For this review, take the finished solid that the model builds, in its own axes (mm). A direction names the side the tool comes from. Coordinates: 2 decimals unless noted, no trailing zeros. Loops run counter-clockwise (first coordinate to the right, second up) from the corner with the lowest first, then second, coordinate; pieces in that order, holes last.
Autodesk Inventor part; units mm, degrees
sketch "Sketch1" plane through (0, 0, 0) normal (0, 0, 1) x (1, 0, 0)
  line L0 (0, 2.8582) -> (0, -2.8582) construction
  line L1 (-5.7775, 0) -> (5.7775, 0) construction
  line L2 (-18.15, -15.5) -> (18.15, -15.5)
  line L3 (18.15, -15.5) -> (18.15, 15.5)
  line L4 (18.15, 15.5) -> (-18.15, 15.5)
  line L5 (-18.15, 15.5) -> (-18.15, -15.5)
  line L6 (-18.15, -15.5) -> (18.15, 15.5) construction
  line L7 (18.15, -15.5) -> (-18.15, 15.5) construction
  point P0 (0, 0)
  point P1 (0, 0)
  dimension "d0" = 36.3
  dimension "d1" = 31
extrude "Extrusion1" add sketch "Sketch1" along normal blind 2.5
sketch "Sketch2" plane through (0, 0, 2.5) normal (0, 0, 1) x (1, 0, 0)
  line L0 (18.15, -15.5) -> (-18.15, -15.5)
  line L1 (-18.15, -15.5) -> (-18.15, 15.5)
  line L2 (-18.15, 15.5) -> (18.15, 15.5)
  line L3 (18.15, 15.5) -> (18.15, -15.5)
  line L4 (-18.15, 15.5) -> (-16.15, 15.5)
  line L5 (-16.15, 15.5) -> (-16.15, -15.5)
  line L6 (-16.15, -15.5) -> (-18.15, -15.5)
  line L7 (-18.15, -15.5) -> (-18.15, 15.5)
  point P0 (0, 0)
  dimension "d4" = 2
extrude "Extrusion2" add sketch "Sketch2" along normal blind 3.5 contours L0 L1 L2 L5
sketch "Sketch3" plane through (0, 0, 6) normal (0, 0, 1) x (1, 0, 0)
  line L0 (-16.15, 15.5) -> (-16.15, -15.5)
  line L1 (-16.15, -15.5) -> (-18.15, -15.5)
  line L2 (-18.15, -15.5) -> (-18.15, 15.5)
  line L3 (-18.15, 15.5) -> (-16.15, 15.5)
  line L4 (-18.15, 5) -> (11.85, 5)
  line L5 (11.85, 5) -> (11.85, -5)
  line L6 (11.85, -5) -> (-18.15, -5)
  line L7 (-18.15, -5) -> (-18.15, 5)
  line L8 (-25.41, 0) -> (25.41, 0)
  point P0 (0, 0)
  point P1 (-16.15, 5)
  point P2 (-16.15, -5)
  dimension "d7" = 10
  dimension "d8" = 5
  dimension "d9" = 30
extrude "Extrusion3" add sketch "Sketch3" along normal blind 2.5
sketch "Sketch4" plane through (0, 0, 2.5) normal (0, 0, 1) x (1, 0, 0)
  line L0 (-16.15, 15.5) -> (-16.15, -15.5)
  line L1 (18.15, -15.5) -> (-16.15, -15.5)
  line L2 (18.15, 15.5) -> (18.15, -15.5)
  line L3 (-16.15, 15.5) -> (18.15, 15.5)
  line L4 (-18.15, 15.5) -> (-16.15, 15.5)
  line L5 (-18.15, -15.5) -> (-18.15, 15.5)
  line L6 (-16.15, -15.5) -> (-18.15, -15.5)
  line L7 (-16.15, 15.5) -> (11.85, 15.5)
  line L8 (11.85, 15.5) -> (11.85, 13)
  line L9 (11.85, 13) -> (-16.15, 13)
  line L10 (-16.15, 13) -> (-16.15, 15.5)
  line L11 (-16.15, -15.5) -> (11.85, -15.5)
  line L12 (11.85, -15.5) -> (11.85, -13)
  line L13 (11.85, -13) -> (-16.15, -13)
  line L14 (-16.15, -13) -> (-16.15, -15.5)
  point P0 (18.15, 13.5)
  point P1 (11.85, -15.5)
  point P2 (11.85, 15.5)
  dimension "d16" = 2.5
  dimension "d17" = 6.3
  dimension "d18" = 6.3
  dimension "d19" = 2.5
extrude "Extrusion4" add sketch "Sketch4" along normal up to surface (6 mm away) contours L3 L8 L9 L0 | L13 L12 L1 L0
sketch "Sketch5" plane through (0, 0, 2.5) normal (0, 0, 1) x (1, 0, 0)
  line L0 (11.85, 13) -> (-16.15, 13)
  line L1 (-16.15, -13) -> (-16.15, 13)
  line L2 (-16.15, -13) -> (11.85, -13)
  line L3 (11.85, -13) -> (11.85, -15.5)
  line L4 (18.15, -15.5) -> (11.85, -15.5)
  line L5 (18.15, 15.5) -> (18.15, -15.5)
  line L6 (11.85, 15.5) -> (18.15, 15.5)
  line L7 (11.85, 15.5) -> (11.85, 13)
  line L8 (11.85, -15.5) -> (-18.15, -15.5)
  line L9 (-18.15, -15.5) -> (-18.15, 15.5)
  line L10 (-18.15, 15.5) -> (11.85, 15.5)
  line L11 (18.15, -15.5) -> (11.85, -15.5)
  line L12 (11.85, -15.5) -> (11.85, 15.5)
  line L13 (11.85, 15.5) -> (18.15, 15.5)
  line L14 (18.15, 15.5) -> (18.15, -15.5)
  point P0 (0, 0)
extrude "Extrusion5" cut sketch "Sketch5" against normal up to surface (2.5 mm away) contours L7 L6 L5 L4 L3 L12
sketch "Sketch6" plane through (-16.15, -5, 6) normal (1, 0, 0) x (0, 0, -1)
  line L0 (0, 0) -> (-2.5, 0)
  line L1 (-2.5, -8) -> (-2.5, 0)
  line L2 (-2.5, -10.5) -> (-2.5, -8)
  line L3 (6, -10.5) -> (-2.5, -10.5)
  line L4 (6, 20.5) -> (6, -10.5)
  line L5 (-2.5, 20.5) -> (6, 20.5)
  line L6 (-2.5, 18) -> (-2.5, 20.5)
  line L7 (-2.5, 10) -> (-2.5, 18)
  line L8 (-2.5, 0) -> (-2.5, 10)
  line L9 (0, 10) -> (0, 0)
  line L10 (-2.5, 10) -> (0, 10)
  line L11 (-2.5, -8) -> (3.5, -8)
  line L12 (3.5, -8) -> (3.5, 18)
  line L13 (3.5, 18) -> (-2.5, 18)
  line L14 (0, 0) -> (-2.5, 0)
  line L15 (-2.5, 0) -> (-2.5, -8)
  line L16 (-2.5, -8) -> (0, -8)
  line L17 (0, -8) -> (0, 0)
  line L18 (-2.5, 10) -> (-2.5, 18)
  line L19 (0, 10) -> (-2.5, 10)
  line L20 (-2.5, 10) -> (-2.5, 18)
  line L21 (-2.5, 18) -> (0, 18)
  line L22 (0, 18) -> (0, 10)
  point P0 (6, 5)
extrude "Extrusion6" add sketch "Sketch6" along normal blind 5 contours L17 L11 L1 L0 | L10 L7 L13 L22
equation "\"d8\" = 0.5 * d7"
equation "\"d18\" = d17"
equation "\"d19\" = d16"
properties part number "LOLIN C3 Mini Holder" material "S235"
Q1. Consider section A-A (x = -3.5). State the section outline as (y, z) points.
Q2. Consider section D-D (x = -12.75). State the section outline as (y, z) points.
Q3. Wall thickness on probe 1 along Y at (x, z) = (8.5, 6.25); probe 2 along Y at (x, z) = (-3, 5); probe 3 along Z at (x, y) = (-14.5, -1): over which ranges is each line inside the solid? List them lowest first.
Q4. Consider section B-B (z = 7.5). State the section outline as (x, y) points.
Q5. For pin 1 Ø3 at (y, z) = (-8, 7) entering from +X; pin 2 Ø1.5 at (x, y) = (-5, 7.5) entering from +Z, all flat-tipped, find the tip position at first contact; note any pin that passes through.
Q6. Consider section C-C (y = 7.5). State the section outline as (x, z) points, then the cut area to 3 significant figures.
Q7. Machinability: for faces 1 (the face through (0, 5, 7)), 2 (the face through (-3, 15.5, 4)), 3 (the face through (-2, -13, 5)), which of the approach directions +Z, -Z, +X, -X, +Y, -Y give a long, thin tool a straight path to every point of the face, cutting with its end or side? Answer none if there is none.
Q8. The part is to be moulded in two halves that separate along Z. For faces 4 (the face through (-2, 0, 2.5)), 5 (the face through (-11.15, 9, 7)), 6 (the face through (-7, 0, 8.5)), say which applies: +Z half, -Z half, draft (parallel to the pull), parting line (faces both ways), or undercut.
Model answer:
1. outline: (-15.5, 0) - (15.5, 0) - (15.5, 8.5) - (13, 8.5) - (13, 2.5) - (-13, 2.5) - (-13, 8.5) - (-15.5, 8.5) - close; (-5, 6) - (5, 6) - (5, 8.5) - (-5, 8.5) - close
2. outline: (-15.5, 0) - (15.5, 0) - (15.5, 8.5) - (-15.5, 8.5) - close; hole (-13, 2.5) - (13, 2.5) - (13, 6) - (-13, 6) - close
3. probe 1: y = -15.5 to -13, -5 to 5, 13 to 15.5
3. probe 2: y = -15.5 to -13, 13 to 15.5
3. probe 3: z = 0 to 2.5, 6 to 8.5
4. outline: (-18.15, -15.5) - (11.85, -15.5) - (11.85, -13) - (-11.15, -13) - (-11.15, -5) - (11.85, -5) - (11.85, 5) - (-11.15, 5) - (-11.15, 13) - (11.85, 13) - (11.85, 15.5) - (-18.15, 15.5) - close
5. pin 1: stops at x = -11.15
5. pin 2: stops at z = 2.5
6. outline: (-18.15, 0) - (11.85, 0) - (11.85, 2.5) - (-16.15, 2.5) - (-16.15, 6) - (-11.15, 6) - (-11.15, 8.5) - (-18.15, 8.5) - close
6. area: 99.5 mm2
7. face 1: +Z, +X
7. face 2: +Z, -Z, +X, -X, +Y
7. face 3: +X
8. face 4: undercut
8. face 5: draft
8. face 6: +Z half
